Design review of the part built by this model. Coordinates are the model's own, in mm. Face numbers are marked on the shaded views. A direction names the side the tool comes from. Coordinates: 2 decimals unless noted, no trailing zeros. Write each loop counter-clockwise with the first axis right and the second up, starting at its lowest first coordinate (ties: lowest second). Pieces come first, ordered by that corner, then holes. Notation, with made-up numbers: (89.25, -14) - (144.25, -14) arc R25 ccw to (144.25, 22) - close; hole circle Ø1 at (52.5, -7.5). An arc over 180 degrees is marked (long way). Use a Markdown table: item, result.
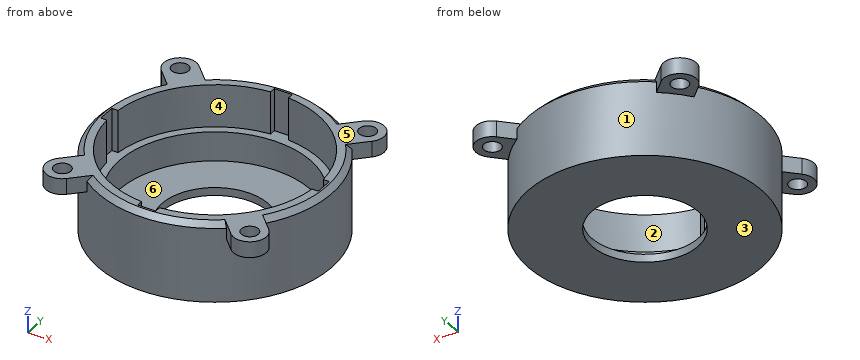
from build123d import *

# Parameters (mm, degrees)
SKETCH1_R               = 22
BOSS_EXTRUDE1_DEPTH     = 8.25
SKETCH2_R               = 18
CUT_EXTRUDE1_DEPTH      = 13.5
SKETCH3_R               = 19.5
CUT_EXTRUDE2_DEPTH      = 8
CUT_EXTRUDE3_DEPTH      = 36.217183306
CUT_EXTRUDE3_DEPTH_BACK = 36.217183306
SKETCH4_R               = 10
SKETCH6_W               = 3.4
SKETCH6_H               = 2.2
CUT_EXTRUDE5_DEPTH      = 8
CIRPATTERN1_COUNT       = 4
CUT_EXTRUDE6_START      = -1.5
SKETCH7_R               = 22
CUT_EXTRUDE6_DEPTH      = 1.5
CHAMFER1_SIZE           = 1
SKETCH8_R               = 1.6
BOSS_EXTRUDE2_DEPTH     = 3
CIRPATTERN2_COUNT       = 4


with BuildPart() as part:
    # Sketch1 → Boss-Extrude1 (new, symmetric)
    with BuildSketch(Plane.XY):
        Circle(SKETCH1_R)
    extrude(amount=BOSS_EXTRUDE1_DEPTH, both=True)

    # Sketch2 → Cut-Extrude1 (cut)
    with BuildSketch(Plane.XY.offset(8.25)):
        Circle(SKETCH2_R)
    extrude(amount=-CUT_EXTRUDE1_DEPTH, mode=Mode.SUBTRACT)

    # Sketch3 → Cut-Extrude2 (cut)
    with BuildSketch(Plane.XY.offset(8.25)):
        Circle(SKETCH3_R)
    extrude(amount=-CUT_EXTRUDE2_DEPTH, mode=Mode.SUBTRACT)

    # Sketch4 → Cut-Extrude3 (cut, two sides: drawn at the far end of the back side and taken through both)
    with BuildSketch(Plane(origin=(0, 0, -8.25), x_dir=(-1, 0, 0), z_dir=(0, 0, -1)).offset(-CUT_EXTRUDE3_DEPTH_BACK)):
        with Locations(Location((0, 0, 0), (0, 0, 180))):
            Circle(SKETCH4_R)
    extrude(amount=CUT_EXTRUDE3_DEPTH + CUT_EXTRUDE3_DEPTH_BACK, mode=Mode.SUBTRACT)

    # Sketch6 → Cut-Extrude5 (cut)
    with BuildSketch(Plane.XY.offset(8.25)):
        with Locations((0, 19.5)):
            Rectangle(SKETCH6_W, SKETCH6_H)
    cut_extrude5 = extrude(amount=-CUT_EXTRUDE5_DEPTH, mode=Mode.SUBTRACT)

    # CirPattern1: Cut-Extrude5 ×4 about axis
    cirpattern1_axis = Axis((0, 0, 0), (0, 0, 1))
    for i in range(1, CIRPATTERN1_COUNT):
        add(cut_extrude5.rotate(cirpattern1_axis, i * 360 / CIRPATTERN1_COUNT), mode=Mode.SUBTRACT)

    # Sketch7 → Cut-Extrude6 (cut)
    with BuildSketch(Plane(origin=(0, 0, -8.25), x_dir=(-1, 0, 0), z_dir=(0, 0, -1)).offset(CUT_EXTRUDE6_START)):
        Circle(SKETCH7_R)
    extrude(amount=CUT_EXTRUDE6_DEPTH, mode=Mode.SUBTRACT)

    # Chamfer1
    chamfer1_edges = [part.edges().sort_by_distance(p)[0] for p in [
        (-22, 0, 8.25),
    ]]
    chamfer(chamfer1_edges, length=CHAMFER1_SIZE)

    # Sketch8 → Boss-Extrude2 (add)
    with BuildSketch(Plane.XY.offset(8.25)):
        with BuildLine():
            Line((15.556349186, 19.940411229), (12.494527459, 16.878589502))
            Line((12.494527459, 16.878589502), (16.878589502, 12.494527459))
            Line((16.878589502, 12.494527459), (19.940411229, 15.556349186))
            ThreePointArc((19.940411229, 15.556349186), (19.940411229, 19.940411229), (15.556349186, 19.940411229))
        make_face()
        with Locations((17.748380208, 17.748380208)):
            Circle(SKETCH8_R, mode=Mode.SUBTRACT)
    boss_extrude2 = extrude(amount=-BOSS_EXTRUDE2_DEPTH)

    # CirPattern2: Boss-Extrude2 ×4 about axis
    cirpattern2_axis = Axis((0, 0, 0), (0, 0, 1))
    for i in range(1, CIRPATTERN2_COUNT):
        add(boss_extrude2.rotate(cirpattern2_axis, i * 360 / CIRPATTERN2_COUNT))


solid = part.part
(1) For pin 1 (2.5 mm diameter, centred on x = 17.75, y = -17.75, fed in from -Z); pin 2 (6 mm diameter, centred on x = -14.5, z = 1, fed in from +Y) (3 decimals); pin 3 (0.6 mm diameter, centred on x = 20, z = 4.5, fed in from +Y); pin 4 (3 mm diameter, centred on x = -5, z = 6.5, fed in from +Y), all flat-tipped, find the tip position at first contact; note any pin that passes through.
Determined:
| item | result |
|---|---|
| pin 1 | through |
| pin 2 | y = 18.755 |
| pin 3 | y = 9.79 |
| pin 4 | y = 21.72 |
(2) Draft analysis for pull direction Y (two halves, no side actions). For the marked faces 4, 5 and 6, state which applies: +Y half, -Y half, draft (parallel to the pull), parting line (faces both ways), or undercut.
Determined:
| item | result |
|---|---|
| face 4 | undercut |
| face 5 | draft |
| face 6 | undercut |
(3) Take a section at A-A on y = 0. Write out the cut boundary in (x, z).
Determined:
| item | result |
|---|---|
| outline | (-22, -6.75) - (-10, -6.75) - (-10, -5.25) - (-18, -5.25) - (-18, 0.25) - (-20.6, 0.25) - (-20.6, 8.25) - (-21, 8.25) - (-22, 7.25) - close; (10, -6.75) - (22, -6.75) - (22, 7.25) - (21, 8.25) - (20.6, 8.25) - (20.6, 0.25) - (18, 0.25) - (18, -5.25) - (10, -5.25) - close |
(4) Machinability: for the marked faces 1, 2 and 3, which of the approach directions +Z, -Z, +X, -X, +Y, -Y give a long, thin tool a straight path to every point of the face, cutting with its end or side? Answer none if there is none.
Determined:
| item | result |
|---|---|
| face 1 | -Z |
| face 2 | +Z |
| face 3 | -Z, +X, -X, +Y, -Y |
(5) Take a section at D-D on z = -3.5. Write out the cut boundary in (x, y), and give its area (3 significant figures).
Determined:
| item | result |
|---|---|
| outline | circle Ø44 at (0, 0); hole circle Ø36 at (0, 0) |
| area | 503 mm2 |
(6) For L1, parallel to Y at x = 0, z = -3.35; L2, parallel to Y at x = 0, z = -6.4; L3, parallel to X at y = -18, z = 7.75, list the stretches that pass through material, from the lowest coordinate up. Write a range as from..to.
Determined:
| item | result |
|---|---|
| L1 | -22..-18, 18..22 |
| L2 | -22..-10, 10..22 |
| L3 | -20.84..-19.33, -16.17..-13.62, -11.76..-7.5, 7.5..11.76, 13.62..16.17, 19.33..20.84 |
(7) Take a section at C-C on z = 1. Write out the cut boundary in (x, y).
Determined:
| item | result |
|---|---|
| outline | circle Ø44 at (0, 0); hole (-20.6, -1.7) - (-19.43, -1.7) arc R19.5 ccw to (-1.7, -19.43) - (-1.7, -20.6) - (1.7, -20.6) - (1.7, -19.43) arc R19.5 ccw to (19.43, -1.7) - (20.6, -1.7) - (20.6, 1.7) - (19.43, 1.7) arc R19.5 ccw to (1.7, 19.43) - (1.7, 20.6) - (-1.7, 20.6) - (-1.7, 19.43) arc R19.5 ccw to (-19.43, 1.7) - (-20.6, 1.7) - close |
